Part print with two shaded views. Sizes in mm from the minimum x, y, z corner. Coordinates: 2 decimals unless noted, no trailing zeros. Loops run counter-clockwise (first coordinate to the right, second up) from the corner with the lowest first, then second, coordinate; pieces in that order, holes last. Notation, with made-up numbers: (24, -27.75) - (37, -27.75) arc R10 cw to (37, -16.75) - close; hole circle Ø7 at (-20.5, 28). An arc over 180 degrees is marked (long way). Answer as CSV lines item,"result".
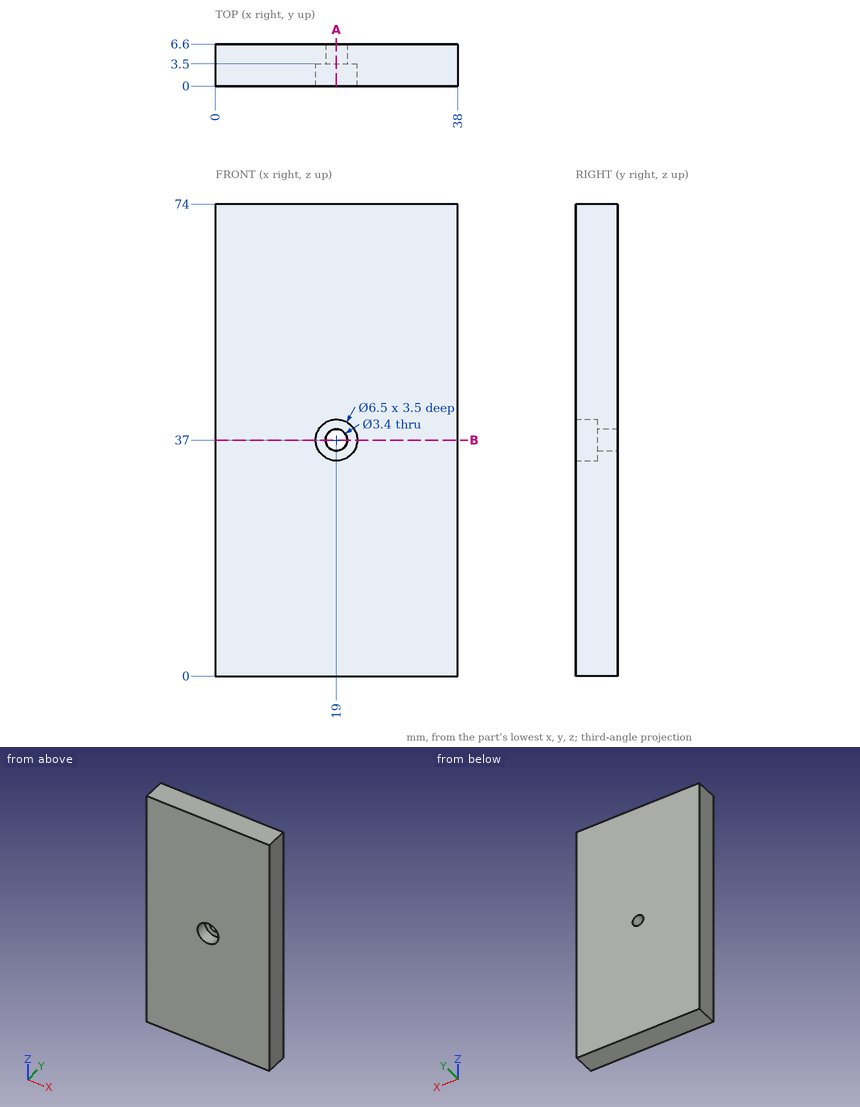
Q1. Flat gauge pin, fed straight in: pin 1 (12 mm diameter, centred on x = 25, z = 62.5, fed in from -Y). Where does the tip first touch, or does it go through?
Results:
pin 1,"stops at y = 0"
Q2. Wall check: L1, parallel to Z at x = 19, y = 2.8; L2, parallel to X at y = 2.6, z = 37; L3, parallel to X at y = 4.9, z = 37. Give the ranges that are in metal, low to high.
Results:
L1,"z = 0 to 33.75, 40.25 to 74"
L2,"x = 0 to 15.75, 22.25 to 38"
L3,"x = 0 to 17.3, 20.7 to 38"
Q3. Saw through at A-A (x = 19). Give the cut face in (y, z).
Results:
outline,"(0, 0) - (6.6, 0) - (6.6, 35.3) - (3.5, 35.3) - (3.5, 33.75) - (0, 33.75) - close; (0, 40.25) - (3.5, 40.25) - (3.5, 38.7) - (6.6, 38.7) - (6.6, 74) - (0, 74) - close"
Q4. Saw through at B-B (z = 37). Give the cut face in (x, y).
Results:
outline,"(0, 0) - (15.75, 0) - (15.75, 3.5) - (17.3, 3.5) - (17.3, 6.6) - (0, 6.6) - close; (20.7, 3.5) - (22.25, 3.5) - (22.25, 0) - (38, 0) - (38, 6.6) - (20.7, 6.6) - close"
